Check sheet for the drawn part. Datum: minimum x, y, z corner. Units: mm. A direction names the side the tool comes from. Round coordinates to 2 decimals unless told otherwise and drop trailing zeros. Write each loop counter-clockwise with the first axis right and the second up, starting at its lowest first coordinate (ties: lowest second). Pieces come first, ordered by that corner, then holes. Notation, with made-up numbers: M -13.5,27 L -6.5,27 A6 cw -6.5,32 Z; hole C 79,73 d11. An arc over 180 degrees is marked long. One line per item, written item: value.
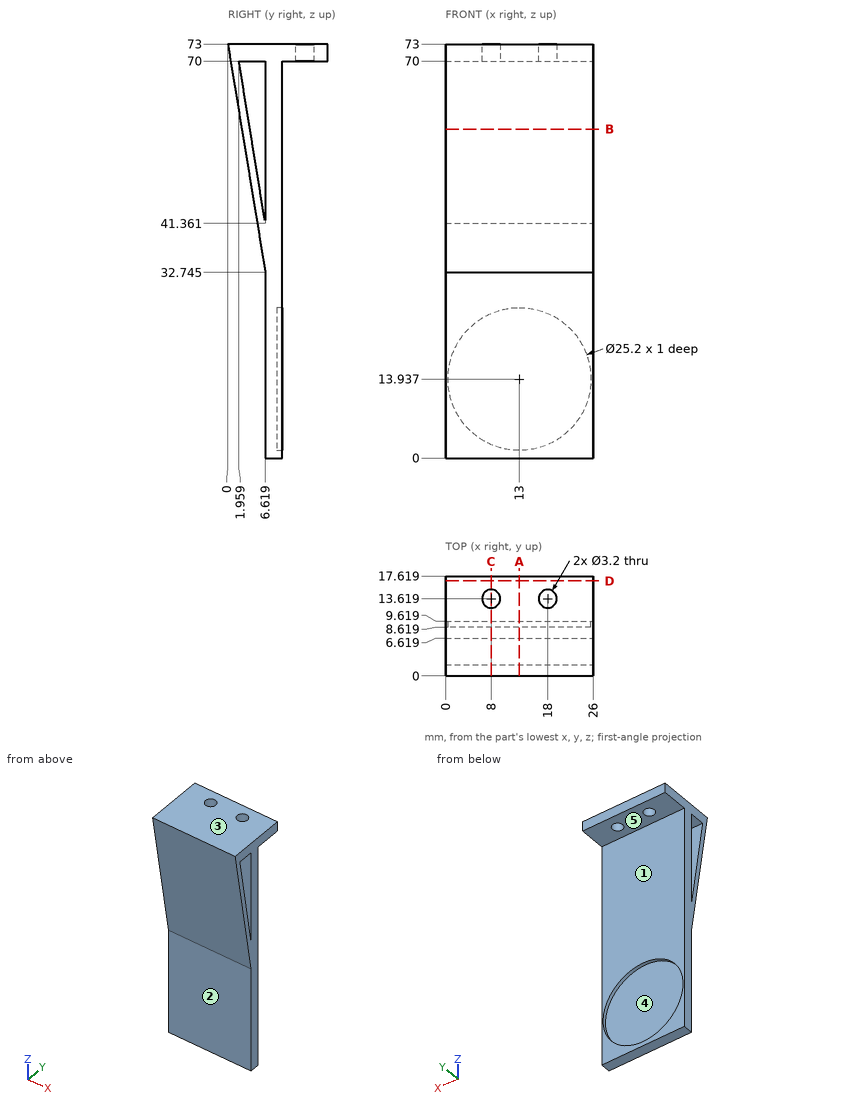
Q1. Sectioned sample at C-C on x = 8. Enter the section's corners in (y, z) (1 decimal), and give its area (3 significant figures).
Completed:
outline: M 0,73 L 6.6,32.7 L 6.6,0 L 9.6,0 L 9.6,2.4 L 8.6,2.4 L 8.6,25.5 L 9.6,25.5 L 9.6,70 L 12,70 L 12,73 Z; M 15.2,70 L 17.6,70 L 17.6,73 L 15.2,73 Z; hole M 2,70 L 6.6,41.4 L 6.6,70 Z
area: 277 mm^2
Q2. Scan lines: line 1 (Y direction, x = 11.25, z = 23); line 2 (Y direction, x = 1.5, z = 30); line 3 (Y direction, x = 18, z = 71.1). Record each from-to range of solid material in increasing order. Write a range as [from, to].
Completed:
line 1: [6.62, 8.62]
line 2: [6.62, 9.62]
line 3: [0.31, 12.02], [15.22, 17.62]
Q3. Depth check by flat-ended pin: P1, Ø9, axis at x = 14.5, y = 13.5, coming from the -Z side; P2, Ø4, axis at x = 18, y = 13.62, coming from the -Z side; P3, Ø7.5, axis at x = 7.5, z = 8, coming from the +Y side; P4, Ø10, axis at x = 13, z = 53.5, coming from the +Y side. Enter the tip coordinate at first touch or a pass-through.
Completed:
P1: z = 0
P2: z = 70
P3: y = 8.62
P4: y = 9.62
Q4. Access from +Z, -Z, +X, -X, +Y, -Y to the whole of each face (thin tool, end or side, straight path). Record for the marked faces 1 and 2.
Completed:
face 1: -Z, +X, -X, +Y
face 2: -Z, +X, -X, -Y
Q5. Draft check along Z on the marked faces 3, 4 and 5. Enter one of: pulls with the +Z half, pulls with the -Z half, needs draft (parallel to the pull), parting line crosses it, or undercut.
Completed:
face 3: pulls with the +Z half
face 4: undercut
face 5: pulls with the -Z half
Q6. Sectioned sample at A-A on x = 13. Enter the section's corners in (y, z) (1 decimal), and give its area (3 significant figures).
Completed:
outline: M 0,73 L 6.6,32.7 L 6.6,0 L 9.6,0 L 9.6,1.3 L 8.6,1.3 L 8.6,26.5 L 9.6,26.5 L 9.6,70 L 17.6,70 L 17.6,73 Z; hole M 2,70 L 6.6,41.4 L 6.6,70 Z
area: 284 mm^2
Q7. Sectioned sample at B-B on z = 58. Enter the section's corners in (x, y).
Completed:
outline: M 0,2.47 L 26,2.47 L 26,3.91 L 0,3.91 Z; M 0,6.62 L 26,6.62 L 26,9.62 L 0,9.62 Z
Q8. Sectioned sample at D-D on y = 16.75. Enter the section's corners in (x, z), and give its area (3 significant figures).
Completed:
outline: M 0,70 L 26,70 L 26,73 L 0,73 Z
area: 78.0 mm^2
